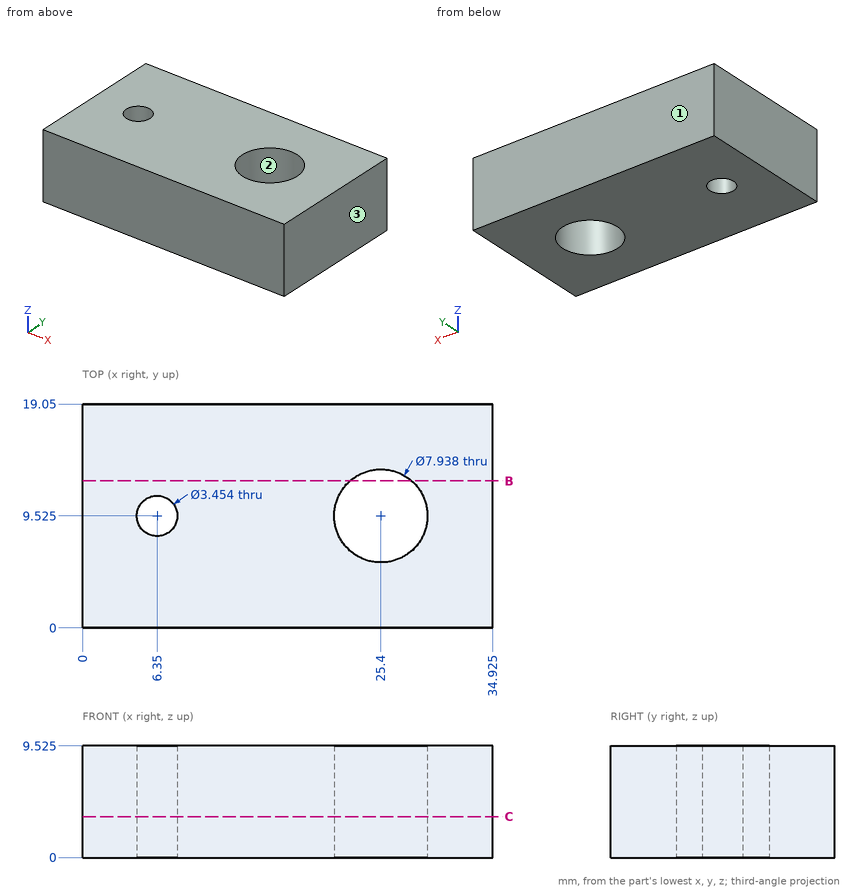
Verification items for this drawing (mm, ordinates from the low corner). Round coordinates to 2 decimals unless told otherwise and drop trailing zeros. Loops run counter-clockwise (first coordinate to the right, second up) from the corner with the lowest first, then second, coordinate; pieces in that order, holes last. Notation, with made-up numbers: (22, 81.5) - (56, 81.5) arc R26 ccw to (56, 114.5) - close; hole circle Ø10 at (58, -22). An arc over 180 degrees is marked (long way). Answer as CSV lines item,"result". Start each with the question number.
Item 1: Section check C-C (z = 3.5). Count the separate pieces of the cut face and the enclosed holes in it.
Item 2: Scan lines: line 1 (Y direction, x = 25.4, z = 3.25); line 2 (X direction, y = 8.5, z = 3.25) (1 decimal); line 3 (X direction, y = 8.75, z = 1.5) (1 decimal). Record each from-to range of solid material in increasing order. Write a range as [from, to].
Item 3: Release check for a two-part mould opening along Y. For the marked faces 1, 2 and 3 record: +Y half, -Y half, draft (parallel to the pull), parting line (faces both ways), or undercut.
Item 4: Section check B-B (y = 12.5). Record the boundary of the cut face in (x, z) (1 decimal), and give its area (3 significant figures).
Report:
1,separate pieces,"1"
1,enclosed holes,"2"
2,line 1,"y = [0, 5.56], [13.49, 19.05]"
2,line 2,"x = [0, 5], [7.7, 21.6], [29.2, 34.9]"
2,line 3,"x = [0, 4.8], [7.9, 21.5], [29.3, 34.9]"
3,face 1,"+Y half"
3,face 2,"undercut"
3,face 3,"draft"
4,outline,"(0, 0) - (22.8, 0) - (22.8, 9.5) - (0, 9.5) - close; (28, 0) - (34.9, 0) - (34.9, 9.5) - (28, 9.5) - close"
4,area,"283 mm2"
